Can you work these out from the model? Positions are in its coordinate system, mm. A direction names the side the tool comes from. Coordinates: 2 decimals unless noted, no trailing zeros. Loops run counter-clockwise (first coordinate to the right, second up) from the corner with the lowest first, then second, coordinate; pieces in that order, holes last.
```python
from build123d import *

# Parameters (mm, degrees)
SKETCH1_W           = 232.0036
SKETCH1_H           = 152.4
BOSS_EXTRUDE1_DEPTH = 3.4036
SKETCH2_R           = 3.4417
SKETCH2_W           = 71.374
SKETCH2_H           = 26.6446
SKETCH2_W_2         = 71.628
CUT_EXTRUDE1_DEPTH  = 278.602260268
SKETCH3_W           = 34.1376
SKETCH3_H           = 13.97
BOSS_EXTRUDE2_DEPTH = 13.97
SKETCH4_W           = 27.5844
SKETCH4_H           = 6.6548
CUT_EXTRUDE2_DEPTH  = 16.51
SKETCH5_W           = 34.1376
SKETCH5_H           = 3.4036
BOSS_EXTRUDE3_DEPTH = 24.13
SKETCH6_W           = 8.382
SKETCH6_H           = 8.382
CUT_EXTRUDE3_DEPTH  = 293.04512201


with BuildPart() as part:
    # Sketch1 → Boss-Extrude1 (new body)
    with BuildSketch(Plane(origin=(0, 0, 0), x_dir=(1, 0, 0), z_dir=(0, 1, 0))):
        with Locations((116.0018, 76.2)):
            Rectangle(SKETCH1_W, SKETCH1_H)
    extrude(amount=BOSS_EXTRUDE1_DEPTH)

    # Sketch2 → Cut-Extrude1 (cut, through all)
    with BuildSketch(Plane(origin=(0, 3.4036, 0), x_dir=(1, 0, 0), z_dir=(0, 1, 0))):
        with Locations(Location((38.1, 120.65, 0), (0, 0, 270))):
            Circle(SKETCH2_R)
        with Locations(Location((38.1, 76.2, 0), (0, 0, 270))):
            Circle(SKETCH2_R)
        with Locations(Location((38.1, 31.75, 0), (0, 0, 270))):
            Circle(SKETCH2_R)
        with Locations((124.587, 120.5357)):
            Rectangle(SKETCH2_W, SKETCH2_H)
        with Locations((124.714, 76.0857)):
            Rectangle(SKETCH2_W_2, SKETCH2_H)
        with Locations((124.714, 31.6357)):
            Rectangle(SKETCH2_W_2, SKETCH2_H)
    extrude(amount=-CUT_EXTRUDE1_DEPTH, mode=Mode.SUBTRACT)

    # Sketch3 → Boss-Extrude2 (add)
    with BuildSketch(Plane.XZ):
        with Locations((116.0907, -149.225)):
            Rectangle(SKETCH3_W, SKETCH3_H)
    extrude(amount=BOSS_EXTRUDE2_DEPTH)

    # Sketch4 → Cut-Extrude2 (cut)
    with BuildSketch(Plane(origin=(0, 0, -156.21), x_dir=(-1, 0, 0), z_dir=(0, 0, -1))):
        with Locations((-115.9637, -6.731)):
            Rectangle(SKETCH4_W, SKETCH4_H)
    extrude(amount=-CUT_EXTRUDE2_DEPTH, mode=Mode.SUBTRACT)

    # Sketch5 → Boss-Extrude3 (add)
    with BuildSketch(Plane(origin=(0, 0, -152.4), x_dir=(-1, 0, 0), z_dir=(0, 0, -1))):
        with Locations((-116.0907, 1.7018)):
            Rectangle(SKETCH5_W, SKETCH5_H)
    extrude(amount=BOSS_EXTRUDE3_DEPTH)

    # Sketch6 → Cut-Extrude3 (cut, through all)
    with BuildSketch(Plane(origin=(0, 3.4036, 0), x_dir=(1, 0, 0), z_dir=(0, 1, 0))):
        with Locations((116.2685, 166.497)):
            Rectangle(SKETCH6_W, SKETCH6_H)
    extrude(amount=-CUT_EXTRUDE3_DEPTH, mode=Mode.SUBTRACT)


solid = part.part
```
Item 1: On a 3-axis mill with a long thin cutter (end or side, diameter ignored), from which of +Z, -Z, +X, -X, +Y, -Y can I reach the whole of each face in a straight line? I mean faces 4 (the face through (118, 3.404, -48)), 5 (the face through (116, -10.058, -149)), 6 (the face through (116, 0, -171)), 7 (the face through (116, -2, -142.24)). Say none if no direction works.
Results are:
face 4: +Z, -Z, +X, -X, +Y
face 5: +Z, -Z
face 6: -Z, +X, -X, -Y
face 7: +Z, +X, -X, -Y
Item 2: Suppose I cut it at A-A, the plane z = -31.75. Please give me the cut outline in (x, y).
Results are:
outline: (0, 0) - (34.66, 0) - (34.66, 3.4) - (0, 3.4) - close; (41.54, 0) - (88.9, 0) - (88.9, 3.4) - (41.54, 3.4) - close; (160.53, 0) - (232, 0) - (232, 3.4) - (160.53, 3.4) - close
Item 3: We'd pull the mould along Z, two halves only. Please class faces 1 (the face through (116, -2, -156.21)), 2 (the face through (38.25, 1.73, -79.64)), 3 (the face through (102.172, -7, -149)): +Z half, -Z half, draft (parallel to the pull), parting line (faces both ways), or undercut.
Results are:
face 1: -Z half
face 2: undercut
face 3: draft
Item 4: I'm going to push flat-ended pins straight in: P1, Ø2.5, axis at y = 2, z = -165, coming from the -X side; P2, Ø1.5, axis at x = 102, y = -4.5, coming from the -Z side; P3, Ø6, axis at x = 123.5, z = -163, coming from the -Y side; P4, Ø1.7, axis at y = 1, z = -29, coming from the -X side. Where does each tip first touch, or does it pass through?
Results are:
P1: stops at x = 99.02
P2: stops at z = -156.21
P3: stops at y = 0
P4: stops at x = 0
Item 5: Suppose I cut it at D-D, the plane z = -120.65. Please give me the cut outline in (x, y), plus the area to 3 significant figures.
Results are:
outline: (0, 0) - (34.66, 0) - (34.66, 3.4) - (0, 3.4) - close; (41.54, 0) - (88.9, 0) - (88.9, 3.4) - (41.54, 3.4) - close; (160.27, 0) - (232, 0) - (232, 3.4) - (160.27, 3.4) - close
area: 523 mm2
Item 6: I need wall thicknesses on line 1 along X through (y, z) = (2.5, -76.2); line 2 along Y through (x, z) = (219.5, -22); line 3 along Z through (x, y) = (130, -3.75). Which ranges of each line are inside material? Lowest first, please.
Results are:
line 1: x = 0 to 34.66, 41.54 to 88.9, 160.53 to 232
line 2: y = 0 to 3.4
line 3: z = -156.21 to -142.24
Item 7: Suppose I cut it at B-B, the plane y = -7. Please give me the cut outline in (x, z), plus the area to 3 significant figures.
Results are:
outline: (99.02, -156.21) - (102.17, -156.21) - (102.17, -142.24) - (99.02, -142.24) - close; (129.76, -156.21) - (133.16, -156.21) - (133.16, -142.24) - (129.76, -142.24) - close
area: 91.5 mm2
Item 8: Suppose I cut it at C-C, the plane x = 148.5. Please give me the cut outline in (y, z).
Results are:
outline: (0, -152.4) - (3.4, -152.4) - (3.4, -133.86) - (0, -133.86) - close; (0, -107.21) - (3.4, -107.21) - (3.4, -89.41) - (0, -89.41) - close; (0, -62.76) - (3.4, -62.76) - (3.4, -44.96) - (0, -44.96) - close; (0, -18.31) - (3.4, -18.31) - (3.4, 0) - (0, 0) - close
